Geometry: final body of the model. Coordinates: model frame, mm. A direction names the side the tool comes from. Give positions to 0.01 mm unless a question says otherwise; leave off trailing zeros. Order: outer loops, then holes, each group sorted by start corner. A loop starts at its lowest first (then second) coordinate and runs counter-clockwise, first axis right, second up. Notation, with made-up numbers: M 38.5,22.25 L 47.5,22.25 A20 cw 47.5,26.25 Z; hole C 23,-25.75 d8. An arc over 180 degrees is marked long. Use CSV: the item, a comma, the result in double quotes.
```python
from build123d import *

# Parameters (mm, degrees)
SKETCH1_R           = 3.05
BOSS_EXTRUDE1_DEPTH = 3
BOSS_EXTRUDE2_DEPTH = 3
FILLET1_R           = 1


# Read off the part's stored shape, not the designer's step: Boss-Extrude2
with BuildPart() as part:
    # Sketch1 → Boss-Extrude1 (new body)
    with BuildSketch(Plane(origin=(0, 0, 0), x_dir=(1, 0, 0), z_dir=(0, 1, 0))):
        with BuildLine():
            Line((0, 6), (40, 6))
            Line((40, 6), (51.329332784, 6))
            Line((51.329332784, 6), (49.031195671, 1.854050901))
            Line((49.031195671, 1.854050901), (51.655054793, 0.39962204))
            Line((51.655054793, 0.39962204), (45.83733935, -10.095814445))
            Line((45.83733935, -10.095814445), (43.213480228, -8.641385585))
            Line((43.213480228, -8.641385585), (40.915343116, -12.787334683))
            Line((40.915343116, -12.787334683), (36.674145691, -6))
            Line((36.674145691, -6), (0, -6))
            ThreePointArc((0, -6), (-6, 0), (0, 6))
        make_face()
        with Locations(Location((0, 0, 0), (0, 0, 270))):
            Circle(SKETCH1_R, mode=Mode.SUBTRACT)
        with Locations(Location((40, 0, 0), (0, 0, 270))):
            Circle(SKETCH1_R, mode=Mode.SUBTRACT)
    extrude(amount=BOSS_EXTRUDE1_DEPTH)

    # Boss-Extrude2 outline → Boss-Extrude2 (add)
    with BuildSketch(Plane(origin=(0, 0, 0), x_dir=(1, 0, 0), z_dir=(0, 1, 0))):
        with BuildLine():
            Line((15.172439685, -59.228761833), (21.596230146, -47.639937071))
            Line((21.596230146, -47.639937071), (6.440532496, -6))
            Line((6.440532496, -6), (0, -6))
            ThreePointArc((0, -6), (-3.441458618, -4.914912266), (-5.638155725, -2.05212086))
            Line((-5.638155725, -2.05212086), (15.172439685, -59.228761833))
        make_face()
    extrude(amount=BOSS_EXTRUDE2_DEPTH)

    # Fillet1
    fillet1_edges = [part.edges().sort_by_distance(p)[0] for p in [
        (51.329332784, 1.5, -6),
        (49.031195671, 1.5, -1.854050901),
        (51.655054793, 1.5, -0.39962204),
        (45.83733935, 1.5, 10.095814445),
        (43.213480228, 1.5, 8.641385585),
        (40.915343116, 1.5, 12.787334683),
        (6.440532496, 1.5, 6),
        (21.596230146, 1.5, 47.639937071),
        (15.172439685, 1.5, 59.228761833),
    ]]
    fillet(fillet1_edges, radius=FILLET1_R)


solid = part.part
```
1. Section A-A, the plane y = 1.7. Return the cut outline in (x, z) (3 decimals).
Answer:
outline,"M -5.638,2.052 A6 ccw 0,-6 L 49.632,-6 A1 ccw 50.506,-4.515 L 49.516,-2.729 A1 cw 49.906,-1.369 L 50.78,-0.884 A1 ccw 51.17,0.475 L 46.322,9.221 A1 ccw 44.963,9.611 L 44.088,9.126 A1 cw 42.729,9.516 L 41.738,11.303 A1 ccw 40.016,11.348 L 36.674,6 L 7.869,6 A1 cw 6.929,7.342 L 21.44,47.212 A1 ccw 21.375,48.039 L 16.236,57.31 A1 ccw 14.422,57.167 Z; hole C 0,0 d6.1; hole C 40,0 d6.1"
2. Section C-C, the plane x = 24.5. Return the cut outline in (y, z), plus the area to 3 significant figures.
Answer:
outline,"M 0,-6 L 3,-6 L 3,6 L 0,6 Z"
area,"36.0 mm2"
3. Pull-direction query (Z, two-part tool) for faces 4 (the face through (40.875, 1.521, 11.818)), 5 (the face through (-4.961, 1.479, -3.375)), 6 (the face through (22, 1, 6)), 7 (the face through (50.5, 1.5, -5.5)); classes: +Z half, -Z half, draft (parallel to the pull), parting line (faces both ways), or undercut.
Answer:
face 4,"+Z half"
face 5,"parting line"
face 6,"undercut"
face 7,"undercut"
4. Section B-B, the plane x = 11. Return the cut outline in (y, z), plus the area to 3 significant figures.
Answer:
outline,"M 0,-6 L 3,-6 L 3,6 L 0,6 Z; M 0,18.53 L 3,18.53 L 3,47.77 L 0,47.77 Z"
area,"124 mm2"
5. Line query: line 1 (X direction, y = 1.6, z = 0); line 2 (Z direction, x = 36.5, y = 0.6); line 3 (X direction, y = 2.3, z = -2.5). Output: solid intervals per line, ascending.
Answer:
line 1,"-6 to -3.05, 3.05 to 36.95, 43.05 to 51.3"
line 2,"-6 to 6"
line 3,"-5.45 to -1.75, 1.75 to 38.25, 41.75 to 49.42"
6. Section D-D, the plane z = 15.5. Return the cut outline in (x, y), plus the area to 3 significant figures.
Answer:
outline,"M -0.74,0 L 9.9,0 L 9.9,3 L -0.74,3 Z"
area,"31.9 mm2"
7. Pin query (flat end, axial travel): pin 1 Ø5.5 at (x, z) = (0, 0) entering from -Y (3 decimals). Return the tip coordinate at first contact, or that it passes through.
Answer:
pin 1,"through"
8. Reachability of faces 1 (the face through (16, 3, 4)), 2 (the face through (38.368, 1.479, 8.711)), 3 (the face through (7.04, 1.52, 6.44)) from +Z, -Z, +X, -X, +Y, -Y: full face, straight path, thin tool, end or side. Return the list, or none.
Answer:
face 1,"+Z, -Z, +X, -X, +Y"
face 2,"+Z, +Y, -Y"
face 3,"+Y, -Y"
